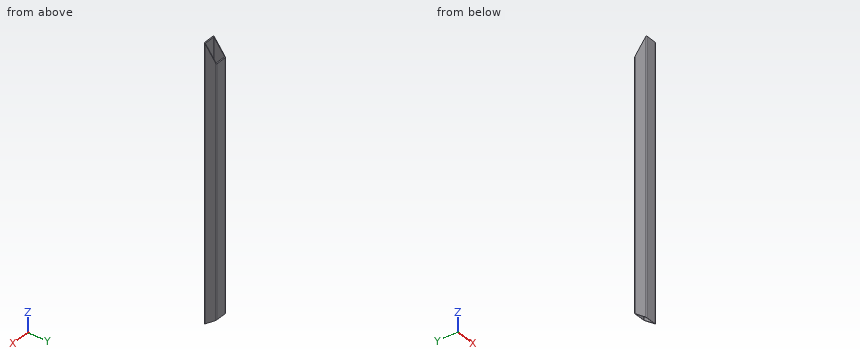
from build123d import *

# Parameters (mm, degrees)
BOSS_EXTRUDE1_DEPTH      = 364.5
BOSS_EXTRUDE1_DEPTH_BACK = 364.5
CUT_EXTRUDE1_DEPTH       = 33
CUT_EXTRUDE2_DEPTH       = 33


with BuildPart() as part:
    # Sketch1 → Boss-Extrude1 (new body, two sides)
    with BuildSketch(Plane.XY) as boss_extrude1_sk:
        with BuildLine():
            Line((-14, -16), (14, -16))
            ThreePointArc((14, -16), (15.414213562, -15.414213562), (16, -14))
            Line((16, -14), (16, 14))
            ThreePointArc((16, 14), (15.414213562, 15.414213562), (14, 16))
            Line((14, 16), (-14, 16))
            ThreePointArc((-14, 16), (-15.414213562, 15.414213562), (-16, 14))
            Line((-16, 14), (-16, -14))
            ThreePointArc((-16, -14), (-15.414213562, -15.414213562), (-14, -16))
        make_face()
        with BuildLine():
            Line((-14, 14.48), (14, 14.48))
            ThreePointArc((14, 14.48), (14.339411255, 14.339411255), (14.48, 14))
            Line((14.48, 14), (14.48, -14))
            ThreePointArc((14.48, -14), (14.339411255, -14.339411255), (14, -14.48))
            Line((14, -14.48), (-14, -14.48))
            ThreePointArc((-14, -14.48), (-14.339411255, -14.339411255), (-14.48, -14))
            Line((-14.48, -14), (-14.48, 14))
            ThreePointArc((-14.48, 14), (-14.339411255, 14.339411255), (-14, 14.48))
        make_face(mode=Mode.SUBTRACT)
    extrude(amount=BOSS_EXTRUDE1_DEPTH)
    extrude(boss_extrude1_sk.sketch, amount=-BOSS_EXTRUDE1_DEPTH_BACK)

    # Sketch2 → Cut-Extrude1 (cut, through all)
    with BuildSketch(Plane(origin=(16, 0, 0), x_dir=(0, 0, -1), z_dir=(1, 0, 0))):
        Polygon((-364.5, -16), (-364.5, 16), (-322.219100301, 16), align=None)
    extrude(amount=-CUT_EXTRUDE1_DEPTH, mode=Mode.SUBTRACT)

    # Sketch3 → Cut-Extrude2 (cut, through all)
    with BuildSketch(Plane(origin=(16, 0, 0), x_dir=(0, 0, -1), z_dir=(1, 0, 0))):
        Polygon((364.5, 16), (364.5, -16), (340.281026249, 16), align=None)
    extrude(amount=-CUT_EXTRUDE2_DEPTH, mode=Mode.SUBTRACT)


solid = part.part
Source: CAD feature listing. Evaluate the final solid. Frame: model axes, mm. Give positions to 0.01 mm unless a question says otherwise; leave off trailing zeros. Write each loop counter-clockwise with the first axis right and the second up, starting at its lowest first coordinate (ties: lowest second). Pieces come first, ordered by that corner, then holes. Notation, with made-up numbers: M 83,50.25 L 128,50.25 A22 ccw 128,88.25 Z; hole C -2,37.25 d11. An arc over 180 degrees is marked long. Return JSON: item names as keys, results as strings. Group by question number.
1) First-contact query: pin 1 Ø6 at (x, y) = (-12.5, 1.5) entering from +Z; pin 2 Ø12 at (x, y) = (-2.5, 0.5) entering from +Z. Flat tips, straight axial feed; report the tip coordinate or a pass-through.
2) Cut plane C-C, the plane z = 97.5. Output: boundary loops of the cut face in (x, y).
3) Cut plane B-B, the plane y = 9. Output: boundary loops of the cut face in (x, z), then the cut area to 3 significant figures.
4) Cut plane A-A, the plane x = -2. Output: boundary loops of the cut face in (y, z), then the cut area to 3 significant figures.
5) Ray query, L1, parallel to X at y = 14, z = 27; L2, parallel to Y at x = -11, z = 323. Return the intervals inside material, ascending.
Data:
{
 "1": {"pin 1": "stops at z = 344.36", "pin 2": "passes through"},
 "2": {"outline": "M -16,-14 A2 ccw -14,-16 L 14,-16 A2 ccw 16,-14 L 16,14 A2 ccw 14,16 L -14,16 A2 ccw -16,14 Z; hole M -14.48,-14 A0.48 ccw -14,-14.48 L 14,-14.48 A0.48 ccw 14.48,-14 L 14.48,14 A0.48 ccw 14,14.48 L -14,14.48 A0.48 ccw -14.48,14 Z"},
 "3": {"outline": "M -16,-345.58 L -14.48,-345.58 L -14.48,331.47 L -16,331.47 Z; M 14.48,-345.58 L 16,-345.58 L 16,331.47 L 14.48,331.47 Z", "area": "2,060 mm²"},
 "4": {"outline": "M -16,-364.5 L -14.48,-363.35 L -14.48,362.49 L -16,364.5 Z; M 14.48,-341.43 L 16,-340.28 L 16,322.22 L 14.48,324.23 Z", "area": "2,120 mm²"},
 "5": {"L1": "x = -16 to -14.48, 14.48 to 16", "L2": "y = -16 to -14.48, 14.48 to 15.41"}
}
